Design review of the part built by this model. Coordinates are the model's own, in mm. A direction names the side the tool comes from. Coordinates: 2 decimals unless noted, no trailing zeros. Loops run counter-clockwise (first coordinate to the right, second up) from the corner with the lowest first, then second, coordinate; pieces in that order, holes last. Notation, with made-up numbers: (55.25, -14.75) -> (93.25, -14.75) arc R22 ccw to (93.25, -4.75) -> close; hole circle Ø7 at (15, -12.5). An arc over 180 degrees is marked (long way). Use CSV: the item, a comma, the result in double quotes.
```python
from build123d import *

# Parameters (mm, degrees)
BOSS_EXTRUDE1_DEPTH     = 2.25
BOSS_EXTRUDE2_DEPTH     = 1.5
CUT_EXTRUDE1_DEPTH      = 4.75
CUT_EXTRUDE1_DEPTH_BACK = 4.75
BOSS_EXTRUDE3_START     = 44.5
SKETCH5_W               = 8
SKETCH5_H               = 12.8
BOSS_EXTRUDE3_DEPTH     = 1.5
BOSS_EXTRUDE4_START     = -44.5
SKETCH5_2_W             = 8
SKETCH5_2_H             = 12.8
BOSS_EXTRUDE4_DEPTH     = 1.5
SKETCH6_R               = 1.2
CUT_EXTRUDE3_DEPTH      = 45.5
CUT_EXTRUDE3_DEPTH_BACK = 45.5
FILLET1_R               = 1.5
SKETCH7_W               = 89
SKETCH7_H               = 89
CUT_EXTRUDE4_DEPTH      = 4.75
BOSS_EXTRUDE5_DEPTH     = 3.75
FILLET2_R               = 1.5
M2X0_4_TAPPED_HOLE1_D   = 1.6


with BuildPart() as part:
    # Sketch1 → Boss-Extrude1 (new body, symmetric)
    with BuildSketch(Plane(origin=(0, 0, 0), x_dir=(1, 0, 0), z_dir=(0, 1, 0))):
        Polygon((-25.5, -35.5), (25.5, -35.5), (35.5, -31.5), (35.5, 31.5), (25.5, 35.5), (-25.5, 35.5), (-35.5, 31.5), (-35.5, -31.5), align=None)
    extrude(amount=BOSS_EXTRUDE1_DEPTH, both=True)

    # Sketch2 → Boss-Extrude2 (add)
    with BuildSketch(Plane(origin=(0, 2.25, 0), x_dir=(1, 0, 0), z_dir=(0, 1, 0))):
        Polygon((27.233241632, -44.5), (44.5, -37.593296653), (44.5, 37.593296653), (27.233241632, 44.5), (-27.233241632, 44.5), (-44.5, 37.593296653), (-44.5, -37.593296653), (-27.233241632, -44.5), align=None)
    boss_extrude2 = extrude(amount=BOSS_EXTRUDE2_DEPTH)

    # Mirror1: Boss-Extrude2 across plane
    add(boss_extrude2.mirror(Plane.ZX))

    # Sketch3 → Cut-Extrude1 (cut, two sides)
    with BuildSketch(Plane(origin=(0, 0, 0), x_dir=(1, 0, 0), z_dir=(0, 1, 0))) as cut_extrude1_sk:
        Polygon((-25.211126395, -34), (25.211126395, -34), (34, -30.484450558), (34, 30.484450558), (25.211126395, 34), (-25.211126395, 34), (-34, 30.484450558), (-34, -30.484450558), align=None)
    extrude(amount=CUT_EXTRUDE1_DEPTH, mode=Mode.SUBTRACT)
    extrude(cut_extrude1_sk.sketch, amount=-CUT_EXTRUDE1_DEPTH_BACK, mode=Mode.SUBTRACT)

    # Sketch5 → Boss-Extrude3 (add)
    with BuildSketch(Plane.XY.offset(BOSS_EXTRUDE3_START)):
        with Locations((-22, 10.15)):
            Rectangle(SKETCH5_W, SKETCH5_H)
        with Locations((22, 10.15)):
            Rectangle(SKETCH5_W, SKETCH5_H)
    extrude(amount=-BOSS_EXTRUDE3_DEPTH)

    # Sketch5<2> → Boss-Extrude4 (add)
    with BuildSketch(Plane.XY.offset(BOSS_EXTRUDE4_START)):
        with Locations((-22, 10.15)):
            Rectangle(SKETCH5_2_W, SKETCH5_2_H)
        with Locations((22, 10.15)):
            Rectangle(SKETCH5_2_W, SKETCH5_2_H)
    extrude(amount=BOSS_EXTRUDE4_DEPTH)

    # Sketch6 → Cut-Extrude3 (cut, two sides)
    with BuildSketch(Plane.XY) as cut_extrude3_sk:
        with Locations((-22, 13.85)):
            Circle(SKETCH6_R)
        with Locations((22, 13.85)):
            Circle(SKETCH6_R)
        with Locations((-22, 8.45)):
            Circle(SKETCH6_R)
        with Locations((22, 8.45)):
            Circle(SKETCH6_R)
    extrude(amount=CUT_EXTRUDE3_DEPTH, mode=Mode.SUBTRACT)
    extrude(cut_extrude3_sk.sketch, amount=-CUT_EXTRUDE3_DEPTH_BACK, mode=Mode.SUBTRACT)

    # Fillet1
    fillet1_edges = [part.edges().sort_by_distance(p)[0] for p in [
        (35.5, 0, 31.5),
        (25.5, 0, 35.5),
        (0, 2.25, -35.5),
        (0, -2.25, -35.5),
        (35.5, 2.25, 0),
        (35.5, -2.25, 0),
        (-35.5, 2.25, 0),
        (-35.5, -2.25, 0),
        (0, 2.25, 35.5),
        (0, -2.25, 35.5),
        (-25.5, 0, -35.5),
        (-30.5, 2.25, -33.5),
        (-35.5, 0, -31.5),
        (-30.5, -2.25, -33.5),
        (35.5, 0, -31.5),
        (30.5, 2.25, -33.5),
        (25.5, 0, -35.5),
        (30.5, -2.25, -33.5),
        (30.5, 2.25, 33.5),
        (30.5, -2.25, 33.5),
        (-35.5, 0, 31.5),
        (-30.5, 2.25, 33.5),
        (-25.5, 0, 35.5),
        (-30.5, -2.25, 33.5),
        (-22, 3.75, -43),
        (22, 3.75, -43),
        (-22, 3.75, 43),
        (22, 3.75, 43),
        (26, 3.75, 43.75),
        (-18, 3.75, 43.75),
        (18, 3.75, 43.75),
        (-26, 3.75, 43.75),
        (18, 3.75, -43.75),
        (26, 3.75, -43.75),
        (-26, 3.75, -43.75),
    ]]
    fillet(fillet1_edges, radius=FILLET1_R)

    # Sketch7 → Cut-Extrude4 (cut, through all)
    with BuildSketch(Plane(origin=(0, 0, 0), x_dir=(1, 0, 0), z_dir=(0, 1, 0))):
        Rectangle(SKETCH7_W, SKETCH7_H)
    extrude(amount=-CUT_EXTRUDE4_DEPTH, mode=Mode.SUBTRACT)

    # Sketch8 → Boss-Extrude5 (add)
    with BuildSketch(Plane(origin=(0, 0, 0), x_dir=(1, 0, 0), z_dir=(0, 1, 0))):
        Polygon((-25.211126395, -34), (-34, -30.484450558), (-34, -27.984450558), (-25.211126395, -27.984450558), align=None)
        Polygon((25.211126395, -27.984450558), (25.211126395, -34), (34, -30.484450558), (34, -27.984450558), align=None)
        Polygon((25.211126395, 34), (34, 30.484450558), (34, 27.984450558), (25.211126395, 27.984450558), align=None)
        Polygon((-25.211126395, 27.984450558), (-25.211126395, 34), (-34, 30.484450558), (-34, 27.984450558), align=None)
    extrude(amount=BOSS_EXTRUDE5_DEPTH)

    # Fillet2
    fillet2_edges = [part.edges().sort_by_distance(p)[0] for p in [
        (25.211126395, 1.875, 34),
        (-25.211126395, 1.875, 34),
        (25.211126395, 1.875, -34),
        (-25.211126395, 1.875, -34),
        (-25.211126395, 1.875, 27.984450558),
        (-34, 1.875, 27.984450558),
        (34, 1.875, 27.984450558),
        (25.211126395, 1.875, 27.984450558),
        (34, 1.875, -27.984450558),
        (25.211126395, 1.875, -27.984450558),
        (-34, 1.875, -27.984450558),
        (-25.211126395, 1.875, -27.984450558),
    ]]
    fillet(fillet2_edges, radius=FILLET2_R)

    # M2x0.4 Tapped Hole1 (through all)
    with Locations(Plane(origin=(0, 3.75, 0), x_dir=(1, 0, 0), z_dir=(0, 1, 0))):
        with Locations((-27.711126395, 30.484450558), (27.711126395, 30.484450558), (27.711126395, -30.484450558), (-27.711126395, -30.484450558)):
            Hole(M2X0_4_TAPPED_HOLE1_D / 2)


solid = part.part
```
Item 1: Add section A-A (x = -11.5). Give the boundary of the cut face in (y, z), then the cut area to 3 significant figures.
Checked values:
outline,"(0, -35.5) -> (0.75, -35.5) arc R1.5 cw to (2.25, -37) -> (2.25, -44.5) -> (3.75, -44.5) -> (3.75, -34) -> (0, -34) -> close; (0, 34) -> (3.75, 34) -> (3.75, 44.5) -> (2.25, 44.5) -> (2.25, 37) arc R1.5 cw to (0.75, 35.5) -> (0, 35.5) -> close"
area,"39.2 mm^2"
Item 2: Add section B-B (y = 8.45). State how many separate pieces and enclosed holes the cut face has, then the cut area to 3 significant figures.
Checked values:
separate pieces,"8"
enclosed holes,"0"
area,"33.6 mm^2"
Item 3: Draft analysis for pull direction X (two halves, no side actions). For faces 4 (the face through (30.4, 1.8, 34)), 5 (the face through (-35.987, 3.001, 40.998)), 6 (the face through (21.05, 13.12, 43.74)), state which applies: pulls with the +X half, pulls with the -X half, needs draft (parallel to the pull), parting line crosses it, or undercut.
Checked values:
face 4,"pulls with the +X half"
face 5,"pulls with the -X half"
face 6,"undercut"
Item 4: To check wall thickness, follow line 1 along X through (y, z) = (13.85, 43.6); line 2 along Y through (x, z) = (22, 43.6); line 3 along X through (y, z) = (3, 21). State the ranges of each line that lie inside material, in increasing order.
Checked values:
line 1,"-26 to -23.2, -20.8 to -18, 18 to 20.8, 23.2 to 26"
line 2,"2.25 to 7.25, 9.65 to 12.65, 15.05 to 16.55"
line 3,"-44.5 to -34, 34 to 44.5"
Item 5: Clearance check with flat-ended pins moving along their axes: pin 1 (1.4 mm diameter, centred on x = -22, y = 8.45, fed in from -Z) (3 decimals); pin 2 (6 mm diameter, centred on x = -34.5, y = 5.5, fed in from +Z); pin 3 (1.2 mm diameter, centred on y = 12, z = -43.5, fed in from -X); pin 4 (2.5 mm diameter, centred on x = 27.71, z = 30.48, fed in from +Y). State where each tip first meets the part, or that it passes through.
Checked values:
pin 1,"through"
pin 2,"z = 42.57"
pin 3,"x = -26"
pin 4,"y = 3.75"
Item 6: Add section C-C (z = 17). Give the boundary of the cut face in (x, y).
Checked values:
outline,"(-44.5, 2.25) -> (-37, 2.25) arc R1.5 cw to (-35.5, 0.75) -> (-35.5, 0) -> (-34, 0) -> (-34, 3.75) -> (-44.5, 3.75) -> close; (34, 0) -> (35.5, 0) -> (35.5, 0.75) arc R1.5 cw to (37, 2.25) -> (44.5, 2.25) -> (44.5, 3.75) -> (34, 3.75) -> close"
Item 7: Machinability: for faces 1 (the face through (34, 2, 0)), 2 (the face through (-22, 11, -43)), 3 (the face through (-22.95, 7.72, -43.74)), which of the approach directions +Z, -Z, +X, -X, +Y, -Y give a long, thin tool a straight path to every point of the face, cutting with its end or side? Answer none if there is none.
Checked values:
face 1,"+Y, -Y"
face 2,"+X, -X, +Y"
face 3,"+Z, -Z"
